Design review of the part built by this model. Coordinates are the model's own, in mm. Face numbers are marked on the shaded views. Give positions to 0.01 mm unless a question says otherwise; leave off trailing zeros. Write each loop counter-clockwise with the first axis right and the second up, starting at its lowest first coordinate (ties: lowest second). Pieces come first, ordered by that corner, then holes. Notation, with made-up numbers: (19.25, 14.5) - (29.25, 14.5) arc R23 ccw to (29.25, 34.5) - close; hole circle Ø9 at (-22.5, 58.25). An arc over 180 degrees is marked (long way). Write each question's results on one line, items separated by ' | '. Start each with the question number.
from build123d import *

# Parameters (mm, degrees)
CROQUIS1_R                = 0.25
SALIENTE_EXTRUIR1_DEPTH   = 6
SALIENTE_EXTRUIR1_2_DEPTH = 6
SALIENTE_EXTRUIR1_3_DEPTH = 6
CROQUIS2_W                = 9.525
CROQUIS2_H                = 4.826
SALIENTE_EXTRUIR2_DEPTH   = 9.652
CROQUIS3_W                = 0.381
CROQUIS3_H                = 4.826
SALIENTE_EXTRUIR3_DEPTH   = 0.381
CROQUIS4_W                = 0.381
CROQUIS4_H                = 0.381
CROQUIS4_W_2              = 0.4
CROQUIS4_H_2              = 0.4
SALIENTE_EXTRUIR4_DEPTH   = 0.4
CROQUIS5_R                = 1.0922
SALIENTE_EXTRUIR5_DEPTH   = 1.524
CROQUIS6_W                = 2.512066748
CROQUIS6_H                = 0.526501072
CORTAR_EXTRUIR1_DEPTH     = 0.762


with BuildPart() as part:
    # Croquis1 → Saliente-Extruir1 (new body)
    with BuildSketch(Plane(origin=(0, 0, 0), x_dir=(1, 0, 0), z_dir=(0, 1, 0))):
        with Locations(Location((0, 0, 0), (0, 0, 270))):
            Circle(CROQUIS1_R)
    extrude(amount=SALIENTE_EXTRUIR1_DEPTH)



with BuildPart() as body_2:
    # Croquis1 → Saliente-Extruir1 2 (new body)
    with BuildSketch(Plane(origin=(0, 0, 0), x_dir=(1, 0, 0), z_dir=(0, 1, 0))):
        with Locations(Location((2.54, 0, 0), (0, 0, 270))):
            Circle(CROQUIS1_R)
    extrude(amount=SALIENTE_EXTRUIR1_2_DEPTH)


with BuildPart() as body_3:
    # Croquis1 → Saliente-Extruir1 3 (new body)
    with BuildSketch(Plane(origin=(0, 0, 0), x_dir=(1, 0, 0), z_dir=(0, 1, 0))):
        with Locations(Location((5.08, 0, 0), (0, 0, 270))):
            Circle(CROQUIS1_R)
    extrude(amount=SALIENTE_EXTRUIR1_3_DEPTH)


with BuildPart() as part_1:
    add(part.part)

    add(body_2.part)  # Saliente-Extruir2 merges body 2

    add(body_3.part)  # Saliente-Extruir2 merges body 3
    # Croquis2 → Saliente-Extruir2 (add)
    with BuildSketch(Plane(origin=(0, 0, 0), x_dir=(1, 0, 0), z_dir=(0, 1, 0))):
        with Locations((2.54, 0)):
            Rectangle(CROQUIS2_W, CROQUIS2_H)
    extrude(amount=-SALIENTE_EXTRUIR2_DEPTH)

    # Croquis3 → Saliente-Extruir3 (add)
    with BuildSketch(Plane(origin=(0, 0, 0), x_dir=(1, 0, 0), z_dir=(0, 1, 0))):
        with Locations((-2.032, 0)):
            Rectangle(CROQUIS3_W, CROQUIS3_H)
        with Locations((7.112, 0)):
            Rectangle(CROQUIS3_W, CROQUIS3_H)
    extrude(amount=SALIENTE_EXTRUIR3_DEPTH)

    # Croquis4 → Saliente-Extruir4 (add)
    with BuildSketch(Plane.XY.offset(2.413)):
        with Locations((-2.032, 0.1905)):
            Rectangle(CROQUIS4_W, CROQUIS4_H)
        with Locations((7.112, 0.1905)):
            Rectangle(CROQUIS4_W, CROQUIS4_H)
        with Locations((-2.032, -9.4615)):
            Rectangle(CROQUIS4_W, CROQUIS4_H)
        with Locations((7.1025, -9.452)):
            Rectangle(CROQUIS4_W_2, CROQUIS4_H_2)
    extrude(amount=SALIENTE_EXTRUIR4_DEPTH)

    # Croquis5 → Saliente-Extruir5 (add)
    with BuildSketch(Plane.XZ.offset(9.652)):
        with Locations(Location((6.0325, 0, 0), (0, 0, 90))):
            Circle(CROQUIS5_R)
    extrude(amount=SALIENTE_EXTRUIR5_DEPTH)

    # Croquis6 → Cortar-Extruir1 (cut)
    with BuildSketch(Plane.XZ.offset(11.176)):
        with Locations((6.0325, 0)):
            Rectangle(CROQUIS6_W, CROQUIS6_H)
    extrude(amount=-CORTAR_EXTRUIR1_DEPTH, mode=Mode.SUBTRACT)


solid = part_1.part
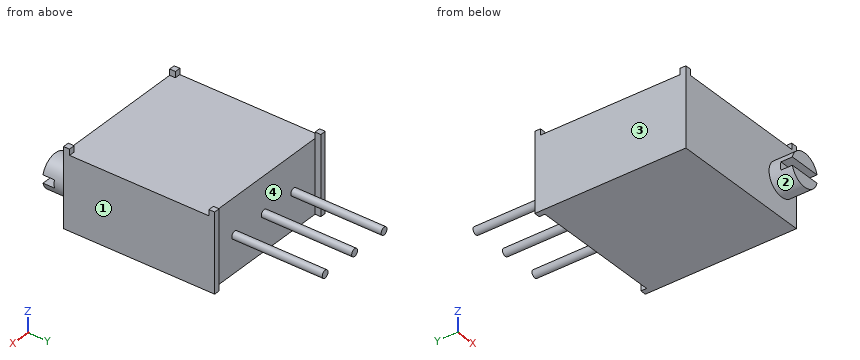
Q1. Add section A-A on z = 0. State the section outline as (x, y) points, plus the area to 3 significant figures.
Q2. The part is to be moulded in two halves that separate along X. For the marked faces 1, 2, 3 and 4, say which applies: +X half, -X half, draft (parallel to the pull), parting line (faces both ways), or undercut.
Q3. Add section D-D on y = -0.25. State the section outline as (x, z) points, plus the area to 3 significant figures.
Q4. Add section B-B on x = 0. State the section outline as (y, z) points, plus the area to 3 significant figures.
Q5. For line 1 along Z through (x, y) = (2.25, -2.75); line 2 along Y through (x, z) = (0.5, -1.2); line 3 along Z through (x, y) = (5.25, 4.75), list the stretches that pass through material, from the lowest coordinate up. Write a range as [from, to].
Q6. Add section C-C on y = 3.25. State the section outline as (x, z) points, plus the area to 3 significant figures.
Q7. Insertion check: P1, Ø0.6, axis at x = 6, y = -11, coming from the -Z side; P2, Ø1.6, axis at x = 2.5, z = -1, coming from the -Y side; P3, Ø1, axis at x = 0, z = 2, coming from the +Y side; P4, Ø1, axis at y = 4, z = -1, coming from the +X side. Each pin has a flat end and moves straight along its axis. Give the tip position at first contact, or say it passes through.
Result:
1) outline: (-2.22, -9.65) - (4.94, -9.65) - (4.94, -10.41) - (7.12, -10.41) - (7.12, -9.65) - (7.3, -9.65) - (7.3, 0.38) - (6.92, 0.38) - (6.92, 0) - (5.33, 0) - (5.33, 6) - (4.83, 6) - (4.83, 0) - (2.79, 0) - (2.79, 6) - (2.29, 6) - (2.29, 0) - (0.25, 0) - (0.25, 6) - (-0.25, 6) - (-0.25, 0) - (-1.84, 0) - (-1.84, 0.38) - (-2.22, 0.38) - close | area: 103 mm²
2) face 1: +X half | face 2: parting line | face 3: -X half | face 4: undercut
3) outline: (-2.22, -2.41) - (7.3, -2.41) - (7.3, 2.41) - (-2.22, 2.41) - close | area: 46.0 mm²
4) outline: (-9.65, -2.41) - (0, -2.41) - (0, -0.25) - (6, -0.25) - (6, 0.25) - (0, 0.25) - (0, 2.41) - (-9.65, 2.41) - close | area: 49.6 mm²
5) line 1: z = [-2.41, 2.41] | line 2: y = [-9.65, 0] | line 3: z = [-0.18, 0.18]
6) outline: circle Ø0.5 at (0, 0); circle Ø0.5 at (2.54, 0); circle Ø0.5 at (5.08, 0) | area: 0.589 mm²
7) P1: stops at z = -1.09 | P2: stops at y = -9.65 | P3: stops at y = 0 | P4: passes through
